```python
from build123d import *

# Parameters (mm, degrees)
SKETCH1_W           = 76.2
SKETCH1_H           = 60.96
BOSS_EXTRUDE1_DEPTH = 12.7
CHAMFER1_SIZE       = 6.35
CUT_EXTRUDE1_DEPTH  = 99.406562789
CRVPATTERN1_DEPTH   = 60.96
SKETCH3_R           = 2.54
CUT_EXTRUDE2_DEPTH  = 5.08


# Read off the part's stored shape, not the designer's step: CrvPattern1
with BuildPart() as part:
    # Sketch1 → Boss-Extrude1 (new body)
    with BuildSketch(Plane(origin=(0, 0, 0), x_dir=(1, 0, 0), z_dir=(0, 1, 0))):
        with Locations((38.1, -30.48)):
            Rectangle(SKETCH1_W, SKETCH1_H)
    extrude(amount=BOSS_EXTRUDE1_DEPTH)

    # Chamfer1
    chamfer1_edges = [part.edges().sort_by_distance(p)[0] for p in [
        (76.2, 12.7, 30.48),
        (38.1, 12.7, 0),
        (0, 12.7, 30.48),
        (38.1, 12.7, 60.96),
    ]]
    chamfer(chamfer1_edges, length=CHAMFER1_SIZE)

    # Sketch2 → Cut-Extrude1 (cut, through all)
    with BuildSketch(Plane.XY.offset(60.96)):
        Polygon((3.048, 0), (5.588, 5.08), (8.128, 0), align=None)
    extrude(amount=-CUT_EXTRUDE1_DEPTH, mode=Mode.SUBTRACT)

    # CrvPattern1 outline → CrvPattern1 (cut)
    with BuildSketch(Plane.XY):
        Polygon((70.612, 5.08), (68.072, 0), (73.152, 0), align=None)
        Polygon((62.484, 5.08), (59.944, 0), (65.024, 0), align=None)
        Polygon((54.356, 5.08), (51.816, 0), (56.896, 0), align=None)
        Polygon((46.228, 5.08), (43.688, 0), (48.768, 0), align=None)
        Polygon((38.1, 5.08), (35.56, 0), (40.64, 0), align=None)
        Polygon((29.972, 5.08), (27.432, 0), (32.512, 0), align=None)
        Polygon((21.844, 5.08), (19.304, 0), (24.384, 0), align=None)
        Polygon((13.716, 5.08), (11.176, 0), (16.256, 0), align=None)
    extrude(amount=CRVPATTERN1_DEPTH, mode=Mode.SUBTRACT)

    # Sketch3 → Cut-Extrude2 (cut)
    with BuildSketch(Plane(origin=(0, 12.7, 0), x_dir=(1, 0, 0), z_dir=(0, 1, 0))):
        with Locations(Location((25.4, -20.32, 0), (0, 0, 270))):
            Circle(SKETCH3_R)
        with Locations(Location((50.8, -20.32, 0), (0, 0, 270))):
            Circle(SKETCH3_R)
        with Locations(Location((25.4, -40.64, 0), (0, 0, 270))):
            Circle(SKETCH3_R)
        with Locations(Location((50.8, -40.64, 0), (0, 0, 270))):
            Circle(SKETCH3_R)
    extrude(amount=-CUT_EXTRUDE2_DEPTH, mode=Mode.SUBTRACT)


solid = part.part
```
CAD build for the part. Positions are in the model's coordinates, mm. A direction names the side the tool comes from. Round coordinates to 2 decimals unless told otherwise and drop trailing zeros. Write each loop counter-clockwise with the first axis right and the second up, starting at its lowest first coordinate (ties: lowest second). Pieces come first, ordered by that corner, then holes.
Item 1: Band-saw the part on A-A on y = 11. Write the cut outline in (x, z), then the cut area to 3 significant figures.
Filled in:
outline: (4.65, 4.65) - (71.55, 4.65) - (71.55, 56.31) - (4.65, 56.31) - close; hole circle Ø5.08 at (25.4, 20.32); hole circle Ø5.08 at (25.4, 40.64); hole circle Ø5.08 at (50.8, 20.32); hole circle Ø5.08 at (50.8, 40.64)
area: 3,370 mm2
Item 2: Tool access for faces 4 (the flat face through (55.644, 2.504, 30.053)), 5 (the flat face through (25, 7.62, 20)), 6 (the flat face through (29, 5, 60.96)): list every direction of +Z, -Z, +X, -X, +Y, -Y with a clear straight run to the whole face (end or side of a thin tool).
Filled in:
face 4: +Z, -Z, -Y
face 5: +Y
face 6: +Z, +X, -X, +Y, -Y
Item 3: Drill centre lines: L1, parallel to X at y = 11.2, z = 40.64; L2, parallel to X at y = 11.6, z = 40.64; L3, parallel to X at y = 9.5, z = 10.5. Where is each one in solid material? Low to high.
Filled in:
L1: x = 4.85 to 22.86, 27.94 to 48.26, 53.34 to 71.35
L2: x = 5.25 to 22.86, 27.94 to 48.26, 53.34 to 70.95
L3: x = 3.15 to 73.05
Item 4: Band-saw the part on C-C on x = 18. Write the cut outline in (y, z).
Filled in:
outline: (0, 0) - (6.35, 0) - (12.7, 6.35) - (12.7, 54.61) - (6.35, 60.96) - (0, 60.96) - close
Item 5: Band-saw the part on D-D on y = 3.25. Give the number of separate pieces and of enclosed holes in the cut face, then the cut area to 3 significant figures.
Filled in:
separate pieces: 10
enclosed holes: 0
area: 3,640 mm2
Item 6: Mould opens along Z. For faces 1 (the cylindrical face through (27.92, 10.2, 19.99)), 2 (the flat face through (37.57, 9.57, 57.74)), 3 (the flat face through (0, 3, 31)) say: released by +Z, released by -Z, zero draft, split by the parting line, or undercut.
Filled in:
face 1: undercut
face 2: released by +Z
face 3: zero draft
Item 7: Drop flat-ended pins along their axis: pin 1 Ø2.5 at (x, z) = (51.5, 40) entering from +Y; pin 2 Ø5 at (x, y) = (65.5, 9) entering from -Z; pin 3 Ø2 at (x, z) = (61, 21.5) entering from -Y. Give the stop position or say it passes through.
Filled in:
pin 1: stops at y = 7.62
pin 2: stops at z = 0.15
pin 3: stops at y = 0.11
